Build history of the part. All positions in model axes, mm. A direction names the side the tool comes from. Round coordinates to 2 decimals unless told otherwise and drop trailing zeros. Order: outer loops, then holes, each group sorted by start corner. A loop starts at its lowest first (then second) coordinate and runs counter-clockwise, first axis right, second up. Notation, with made-up numbers: (28, 20) -> (66, 20) arc R26 cw to (66, 48) -> close; hole circle Ø6 at (61.5, 76). An arc over 180 degrees is marked (long way). Use a Markdown table: item, result. Add a question column.
Item 1: Slice it at C-C, the plane y = -44. Give the cut face in (x, z).
Item 2: Slice it at D-D, the plane x = 21. Give the cut face in (y, z).
Item 3: Slice it at B-B, the plane y = 14. Give the cut face in (x, z), plus the area to 3 significant figures.
Item 4: 3-axis set-ups, long thin cutter, end or side, ignore diameter. For faces 1 (the face through (0.04, 5.66, -12.18)), 2 (the face through (0, 68, 3)), 3 (the face through (0.038, 1.772, -19.978)), 4 (the face through (-16, -48.5, 3)): which of +Z, -Z, +X, -X, +Y, -Y reach the whole face in a straight line?
Item 5: Two-plate mould, pull along X, no slides. Class faces 5 (the face through (-5, -36, 3)), 6 (the face through (-14, 48.5, 3)), 7 (the face through (14.819, 95.996, 2.712)): released by +X, released by -X, zero draft, split by the parting line, or undercut.
Item 6: Pin check, flat tips, straight feed: pin 1 (8 mm diameter, centred on x = 3.5, z = -30.5, fed in from -Y); pin 2 (1.6 mm diameter, centred on y = 66, z = 3, fed in from -X); pin 3 (19 mm diameter, centred on y = -24, z = -31.5, fed in from -X). Stop position of each tip, or through.
Item 7: Slice it at A-A, the plane x = 14.5. Give the cut face in (y, z), plus the area to 3 significant figures.
Item 8: Probe L1, parallel to Y at x = -24.5, z = 3.8; L2, parallel to X at y = -37, z = 0.5; L3, parallel to Z at x = -3, y = 26. List the from-to ranges inside material, lowest first.
from build123d import *

# Parameters (mm, degrees)
F0_R      = 10
F1_DEPTH  = 5.5
F2_R      = 1.5
F3_DEPTH  = 5.5
F4_W      = 5
F4_H      = 24.9248821884
F5_DEPTH  = 5.5
F6_R      = 11.5
F7_DEPTH  = 2.75
F8_R      = 1
F10_DEPTH = 5.5
F11_R     = 1


with BuildPart() as f1:
    # F0 (on Top) → F1 (new body)
    with BuildSketch(Plane.XY):
        with BuildLine():
            Line((-27, -48.5), (27, -48.5))
            ThreePointArc((27, -48.5), (28.4142135624, -47.9142135624), (29, -46.5))
            Line((29, -46.5), (29, 81.5))
            ThreePointArc((29, 81.5), (14.5, 96), (0, 81.5))
            Line((0, 81.5), (0, 53.5))
            ThreePointArc((0, 53.5), (-1.4644660941, 49.9644660941), (-5, 48.5))
            Line((-5, 48.5), (-24, 48.5))
            ThreePointArc((-24, 48.5), (-27.5355339059, 47.0355339059), (-29, 43.5))
            Line((-29, 43.5), (-29, -46.5))
            ThreePointArc((-29, -46.5), (-28.4142135624, -47.9142135624), (-27, -48.5))
        make_face()
        with Locations((14.5, 81.5)):
            Circle(F0_R, mode=Mode.SUBTRACT)
    extrude(amount=F1_DEPTH)

    # F2 (on face) → F3 (cut, through all)
    with BuildSketch(Plane.XY.offset(5.5)):
        with Locations((-24.5, 14)):
            Circle(F2_R)
        with Locations((24.5, 14)):
            Circle(F2_R)
        with Locations((24.5, -44)):
            Circle(F2_R)
        with Locations((-24.5, -44)):
            Circle(F2_R)
    extrude(amount=-F3_DEPTH, mode=Mode.SUBTRACT)

    # F4 (on face) → F5 (cut, through all)
    with BuildSketch(Plane.XY.offset(5.5)):
        with Locations((2.5, -36.0375589058)):
            Rectangle(F4_W, F4_H)
        with Locations((-2.5, -36.0375589058)):
            Rectangle(F4_W, F4_H)
    extrude(amount=-F5_DEPTH, mode=Mode.SUBTRACT)

    # F6 (on Right) → F7 (join, symmetric)
    with BuildSketch(Plane.YZ):
        with BuildLine():
            Line((-49.9737205584, 5.5), (-48.5, 0))
            Line((-48.5, 0), (-32.9708572938, -57.9555495773))
            Line((-32.9708572938, -57.9555495773), (24.6665156112, -1.715730829))
            ThreePointArc((24.6665156112, -1.715730829), (24.8943496088, -0.6229925922), (23.9681393656, 0))
            Line((23.9681393656, 0), (-23.5751178116, 0))
            Line((-23.5751178116, 0), (-23.5751178116, 5.5))
            Line((-23.5751178116, 5.5), (-48.5, 5.5))
            Line((-48.5, 5.5), (-49.9737205584, 5.5))
        make_face()
        with Locations((-23.7671827683, -24.4311470085)):
            Circle(F6_R, mode=Mode.SUBTRACT)
    extrude(amount=F7_DEPTH, both=True)

    # F8
    f8_edges = [f1.edges().sort_by_distance(p)[0] for p in [
        (0, -49.973721, 5.5),
        (0, -32.970857, -57.95555),
    ]]
    fillet(f8_edges, radius=F8_R)

    # F9 (on face) → F10 (cut, through all)
    with BuildSketch(Plane.YZ.offset(2.75)):
        with BuildLine():
            ThreePointArc((-7.9046124855, -17.0336287316), (-7.9432792247, -21.2895926303), (-3.6871553257, -21.3011330035))
            Line((-3.6871553257, -21.3011330035), (-0.2292870065, -17.9271088638))
            Line((-0.2292870065, -17.9271088638), (3.8098796459, -22.0666484241))
            Line((3.8098796459, -22.0666484241), (7.6828757476, -18.2875622549))
            Line((7.6828757476, -18.2875622549), (3.5909387901, -14.1995134591))
            Line((3.5909387901, -14.1995134591), (7.0488071093, -10.8254893195))
            ThreePointArc((7.0488071093, -10.8254893195), (7.0602741622, -6.596406123), (2.8313499495, -6.5579850476))
            Line((2.8313499495, -6.5579850476), (-7.9046124855, -17.0336287316))
        make_face()
    extrude(amount=-F10_DEPTH, mode=Mode.SUBTRACT)

    # F11
    f11_edges = [f1.edges().sort_by_distance(p)[0] for p in [
        (0, -0.229287, -17.927109),
        (0, 3.590939, -14.199513),
        (0, 7.682876, -18.287562),
        (0, 3.80988, -22.066648),
    ]]
    fillet(f11_edges, radius=F11_R)


solid = f1.part
Check sheet entries:
| question | item | result |
|---|---|---|
| 1 | outline | (-29, 0) -> (-26, 0) -> (-26, 5.5) -> (-29, 5.5) -> close; (-23, 0) -> (-5, 0) -> (-5, 5.5) -> (-23, 5.5) -> close; (-2.75, -16.79) -> (2.75, -16.79) -> (2.75, 5.5) -> (-2.75, 5.5) -> close; (5, 0) -> (23, 0) -> (23, 5.5) -> (5, 5.5) -> close; (26, 0) -> (29, 0) -> (29, 5.5) -> (26, 5.5) -> close |
| 2 | outline | (-48.5, 0) -> (73.9, 0) -> (73.9, 5.5) -> (-48.5, 5.5) -> close; (89.1, 0) -> (94.46, 0) -> (94.46, 5.5) -> (89.1, 5.5) -> close |
| 3 | outline | (-29, 0) -> (-26, 0) -> (-26, 5.5) -> (-29, 5.5) -> close; (-23, 0) -> (-2.75, 0) -> (-2.75, -12.12) -> (2.75, -12.12) -> (2.75, 0) -> (23, 0) -> (23, 5.5) -> (-23, 5.5) -> close; (26, 0) -> (29, 0) -> (29, 5.5) -> (26, 5.5) -> close |
| 3 | area | 353 mm2 |
| 4 | face 1 | +X, -X |
| 4 | face 2 | +Z, -Z, -X, +Y |
| 4 | face 3 | +X, -X, +Y |
| 4 | face 4 | +Z, -Z, -X, -Y |
| 5 | face 5 | undercut |
| 5 | face 6 | zero draft |
| 5 | face 7 | split by the parting line |
| 6 | pin 1 | y = -41.38 |
| 6 | pin 2 | x = 0 |
| 6 | pin 3 | x = -2.75 |
| 7 | outline | (-48.5, 0) -> (71.5, 0) -> (71.5, 5.5) -> (-48.5, 5.5) -> close; (91.5, 0) -> (96, 0) -> (96, 5.5) -> (91.5, 5.5) -> close |
| 7 | area | 685 mm2 |
| 8 | L1 | -48.5 to -45.5, -42.5 to 12.5, 15.5 to 48.47 |
| 8 | L2 | -29 to -5, -2.75 to 2.75, 5 to 29 |
| 8 | L3 | 0 to 5.5 |
